Autodesk Inventor part; units mm, degrees
ref_plane "YZ Plane" through (0, 0, 0) normal (1, 0, 0) x (0, 1, 0)
ref_plane "XZ Plane" through (0, 0, 0) normal (0, 1, 0) x (-1, 0, 0)
ref_plane "XY Plane" through (0, 0, 0) normal (0, 0, 1) x (1, 0, 0)
sketch "スケッチ1" plane through (0, 0, 0) normal (0, 0, 1) x (1, 0, 0)
  line L0 (-170, -235) -> (170, -235)
  line L1 (190, -215) -> (190, 215)
  line L2 (170, 235) -> (-170, 235)
  line L3 (-190, 215) -> (-190, -215)
  line L4 (-190, -235) -> (190, 235) construction
  line L5 (190, -235) -> (-190, 235) construction
  circle A0 centre (-180, 225) radius 2.25
  circle A1 centre (180, 225) radius 2.25
  circle A2 centre (-180, -225) radius 2.25
  circle A3 centre (180, -225) radius 2.25
  arc A4 (-170, 235) -> (-190, 215) centre (-170, 215) ccw
  arc A5 (190, 215) -> (170, 235) centre (170, 215) ccw
  arc A6 (170, -235) -> (190, -215) centre (170, -215) ccw
  arc A7 (-190, -215) -> (-170, -235) centre (-170, -215) ccw
  point P0 (0, 0)
  dimension "d0" = 380
  dimension "d1" = 470
  dimension "d2" = 4.5
  dimension "d3" = 10
  dimension "d4" = 10
  dimension "d5" = 10
  dimension "d6" = 10
  dimension "d7" = 10
  dimension "d8" = 10
  dimension "d9" = 10
  dimension "d10" = 10
  dimension "d11" = 20
extrude "押し出し1" add sketch "スケッチ1" along normal blind 3
sketch "スケッチ2" plane through (0, 0, 3) normal (0, 0, 1) x (1, 0, 0)
  circle A0 centre (-180, -225) radius 2.25 construction
  circle A1 centre (-180, -115) radius 2.25
  line L0 (-190, 215) -> (-190, -215)
  point P0 (0, 0)
  dimension "d14" = 110
  dimension "d15" = 10
extrude "押し出し2" cut sketch "スケッチ2" against normal blind 10
sketch "スケッチ3" plane through (0, 0, 3) normal (0, 0, 1) x (1, 0, 0)
  line L0 (-167, -124.6) -> (-167, -215) construction
  line L1 (-170, -124.6) -> (-167, -124.6) construction
  line L2 (-170, -215) -> (-170, -124.6) construction
  line L3 (-170, -215) -> (-167, -215) construction
  line L4 (-170.2, -124.4) -> (-166.8, -124.4)
  line L5 (-166.8, -124.4) -> (-166.8, -215.2)
  line L6 (-166.8, -215.2) -> (-170.2, -215.2)
  line L7 (-170.2, -215.2) -> (-170.2, -124.4)
  point P0 (0, 0)
  dimension "d18" = 0.2
extrude "押し出し3" cut sketch "スケッチ3" against normal up to surface (3 mm away)
sketch "スケッチ4" plane through (0, 0, 3) normal (0, 0, 1) x (1, 0, 0)
  circle A0 centre (-180, -225) radius 2.25 construction
  circle A1 centre (-180, -115) radius 2.25 construction
  circle A2 centre (180, -225) radius 2.25 construction
  circle A3 centre (-180, 225) radius 2.25 construction
  circle A4 centre (180, 225) radius 2.25 construction
  circle A5 centre (-180, -225) radius 2.25 construction
  circle A6 centre (-180, -115) radius 2.25 construction
  circle A7 centre (-180, -225) radius 110 construction
  circle A8 centre (-180, 225) radius 2.25 construction
  circle A9 centre (-180, 225) radius 110 construction
  circle A10 centre (180, 225) radius 110 construction
  circle A11 centre (180, -225) radius 110 construction
  line L0 (-180, -225) -> (180, -225) construction
  line L1 (180, -225) -> (180, 225) construction
  line L2 (180, 225) -> (-180, 225) construction
  line L3 (-180, 225) -> (-180, -225) construction
  line L4 (-180, 0) -> (180, 0) construction
  circle A12 centre (-180, 115) radius 2.25
  circle A13 centre (-180, 0) radius 2.25
  circle A14 centre (-70, -225) radius 2.25
  circle A15 centre (70, -225) radius 2.25
  circle A16 centre (180, -115) radius 2.25
  circle A17 centre (180, 115) radius 2.25
  circle A18 centre (70, 225) radius 2.25
  circle A19 centre (-70, 225) radius 2.25
  circle A20 centre (180, 0) radius 2.25
  point P0 (0, 0)
extrude "押し出し4" cut sketch "スケッチ4" against normal up to surface (3 mm away)
sketch "スケッチ5" plane through (0, 0, 3) normal (0, 0, 1) x (1, 0, 0)
  line L0 (-160, -115) -> (-20, -115) construction
  line L1 (-20, -115) -> (-20, 25) construction
  line L2 (-20, 25) -> (-160, 25) construction
  line L3 (-160, 25) -> (-160, -115) construction
  line L4 (-20, -115) -> (120, -115) construction
  line L5 (120, -115) -> (120, 25) construction
  line L6 (120, 25) -> (-20, 25) construction
  line L7 (-20, 25) -> (-20, -115) construction
  line L8 (-170, -235) -> (170, -235) construction
  line L9 (-190, 215) -> (-190, -215) construction
  line L10 (-152.5, -107.5) -> (-27.5, -107.5) construction
  line L11 (-27.5, -107.5) -> (-27.5, 17.5) construction
  line L12 (-27.5, 17.5) -> (-152.5, 17.5) construction
  line L13 (-152.5, 17.5) -> (-152.5, -107.5) construction
  line L14 (-12.5, 17.5) -> (112.5, 17.5) construction
  line L15 (112.5, 17.5) -> (112.5, -107.5) construction
  line L16 (112.5, -107.5) -> (-12.5, -107.5) construction
  line L17 (-12.5, -107.5) -> (-12.5, 17.5) construction
  circle A0 centre (-152.5, 17.5) radius 2.25
  circle A1 centre (-27.5, 17.5) radius 2.25
  circle A2 centre (-152.5, -107.5) radius 2.25
  circle A3 centre (-27.5, -107.5) radius 2.25
  circle A4 centre (-12.5, -107.5) radius 2.25
  circle A5 centre (-12.5, 17.5) radius 2.25
  circle A6 centre (112.5, 17.5) radius 2.25
  circle A7 centre (112.5, -107.5) radius 2.25
  line L18 (-144, 25) -> (-144, 9)
  line L19 (-144, 9) -> (-160, 9)
  line L20 (-160, 9) -> (-160, -99)
  line L21 (-160, -99) -> (-144, -99)
  line L22 (-144, -99) -> (-144, -115)
  line L23 (-144, -115) -> (-36, -115)
  line L24 (-36, -115) -> (-36, -99)
  line L25 (-36, -99) -> (-4, -99)
  line L26 (-4, -99) -> (-4, -115)
  line L27 (-4, -115) -> (104, -115)
  line L28 (104, -115) -> (104, -99)
  line L29 (104, -99) -> (120, -99)
  line L30 (120, -99) -> (120, 9)
  line L31 (120, 9) -> (104, 9)
  line L32 (104, 9) -> (104, 25)
  line L33 (104, 25) -> (-4, 25)
  line L34 (-4, 25) -> (-4, 9)
  line L35 (-4, 9) -> (-36, 9)
  line L36 (-36, 9) -> (-36, 25)
  line L37 (-36, 25) -> (-144, 25)
  point P0 (0, 0)
  dimension "d23" = 140
  dimension "d24" = 0
  dimension "d25" = 120
  dimension "d26" = 30
  dimension "d27" = 125
  dimension "d28" = 125
  dimension "d29" = 7.5
  dimension "d30" = 7.5
  dimension "d31" = 7.5
  dimension "d32" = 7.5
  dimension "d33" = 7.5
  dimension "d34" = 4.5
  dimension "d35" = 16
  dimension "d36" = 16
extrude "押し出し5" cut sketch "スケッチ5" against normal through all
fillet "フィレット1" radius 8 8 edges at (-144, 9, 1.5) (-144, -99, 1.5) (-36, -99, 1.5) (-4, -99, 1.5) (104, -99, 1.5) (104, 9, 1.5) (-4, 9, 1.5) (-36, 9, 1.5)
fillet "フィレット1" radius 5.3333 12 edges at (-144, 25, 1.5) (-160, 9, 1.5) (-160, -99, 1.5) (-144, -115, 1.5) (-36, -115, 1.5) (-4, -115, 1.5) (104, -115, 1.5) (120, -99, 1.5) (120, 9, 1.5) (104, 25, 1.5) (-4, 25, 1.5) (-36, 25, 1.5)
equation "\"d5\" = d3"
equation "\"d6\" = d4"
equation "\"d7\" = d6"
equation "\"d8\" = d5"
equation "\"d9\" = d8"
equation "\"d10\" = d7"
equation "\"d30\" = d29"
equation "\"d31\" = d30"
equation "\"d32\" = d30"
equation "\"d33\" = d31"
equation "\"d36\" = d35"
equation "\"d39\" = 0.5 * d35"
equation "\"d40\" = 0.333333 * d35"
properties part number "left_panel_amd" material "アルミニウム 6061"
For this review, take the finished solid that the model builds, in its own axes (mm). Coordinates: 2 decimals unless noted, no trailing zeros. Write each loop counter-clockwise with the first axis right and the second up, starting at its lowest first coordinate (ties: lowest second). Pieces come first, ordered by that corner, then holes.
(1) Add section B-B on x = 21. Give the boundary of the cut face in (y, z).
(2) Wall thickness on probe 1 along Y at (x, z) = (-27.5, 2.35); probe 2 along Y at (x, z) = (96, 2.3); probe 3 along Y at (x, z) = (70, 1.45): over which ranges is each line inside the solid? List them lowest first.
(3) Add section C-C on z = 0.8. Count the separate pieces of the cut face and the enclosed holes in it, then the cut area to 3 significant figures.
(4) For pin 1 Ø2.5 at (x, y) = (-152.5, 17.5) entering from -Z; pin 2 Ø5 at (x, y) = (180, 225) entering from +Z, all flat-tipped, find the tip position at first contact; note any pin that passes through.
(5) Add section A-A on y = -66.5. Give the boundary of the cut face in (x, z).
Answer sheet:
1. outline: (-235, 0) - (-115, 0) - (-115, 3) - (-235, 3) - close; (25, 0) - (235, 0) - (235, 3) - (25, 3) - close
2. probe 1: y = -235 to -109.75, -105.25 to -99, 9 to 15.25, 19.75 to 235
2. probe 2: y = -235 to -115, 25 to 235
2. probe 3: y = -235 to -227.25, -222.75 to -115, 25 to 222.75, 227.25 to 235
3. separate pieces: 1
3. enclosed holes: 24
3. area: 140,000 mm2
4. pin 1: passes through
4. pin 2: stops at z = 3
5. outline: (-190, 0) - (-160, 0) - (-160, 3) - (-190, 3) - close; (120, 0) - (190, 0) - (190, 3) - (120, 3) - close
